Autodesk Inventor part; units mm, degrees
ref_plane "YZ Plane" through (0, 0, 0) normal (1, 0, 0) x (0, 1, 0)
ref_plane "XZ Plane" through (0, 0, 0) normal (0, 1, 0) x (-1, 0, 0)
ref_plane "XY Plane" through (0, 0, 0) normal (0, 0, 1) x (1, 0, 0)
sketch "Sketch1" plane through (0, 0, 0) normal (0, 0, 1) x (1, 0, 0)
  line L0 (0, 0) -> (38.1, 0)
  line L1 (38.1, 0) -> (38.1, 253.0348)
  arc A0 (38.1, 507.0348) -> (38.1, 253.0348) centre (666.75, 380.0348) ccw
  line L2 (38.1, 507.0348) -> (38.1, 608.6348)
  line L3 (38.1, 608.6348) -> (0, 608.6348)
  line L4 (0, 608.6348) -> (0, 0)
  circle A1 centre (31.75, 151.4348) radius 3.3655
  circle A2 centre (31.75, 34.671) radius 3.3655
  circle A3 centre (12.7, 12.7) radius 3.3655
  circle A4 centre (12.7, 342.9) radius 3.3655
  circle A5 centre (12.7, 595.9348) radius 3.3655
  circle A6 centre (31.75, 12.7) radius 3.3655
  circle A7 centre (31.75, 253.0348) radius 3.3655
  circle A8 centre (31.75, 507.0348) radius 3.3655
  circle A9 centre (31.75, 595.9348) radius 3.3655
  line L5 (0, 557.8348) -> (0, 608.6348)
  line L6 (0, 50.8) -> (0, 0)
  line L7 (12.7, 342.9) -> (0, 304.3174) construction
  line L8 (0, 317.5) -> (0, 368.3)
  line L9 (0, 129.921) -> (12.7, 129.921) construction
  circle A10 centre (12.7, 129.921) radius 3.3655
  circle A11 centre (12.7, 174.371) radius 3.3655
  line L10 (9.3413, 197.482) -> (9.3413, 204.213)
  line L11 (16.0611, 204.488) -> (16.0611, 197.3435)
  arc A12 (16.0611, 204.488) -> (9.3413, 204.213) centre (12.6956, 204.488) ccw
  arc A13 (9.3413, 197.482) -> (16.0611, 197.3435) centre (12.6974, 197.231) ccw
  circle A14 centre (12.7, 217.188) radius 3.3655
  dimension "d0" = 38.1
  dimension "d2" = 101.6
  dimension "d4" = 457.2
  dimension "d5" = 101.6
  dimension "d6" = 666.75
  dimension "d7" = 641.35
  dimension "d9" = 116.7638
  dimension "d10" = 6.35
  dimension "d11" = 6.35
  dimension "d13" = 12.7
  dimension "d14" = 12.7
  dimension "d16" = 12.7
  dimension "d17" = 342.9
  dimension "d19" = 12.7
  dimension "d20" = 12.7
  dimension "d22" = 6.35
  dimension "d24" = 6.35
  dimension "d25" = 6.731
  dimension "d26" = 6.35
  dimension "hole" = 6.731
  dimension "d28" = 6.35
  dimension "d45" = 12.7
  dimension "d47" = 12.7
  dimension "d54" = 6.731
  dimension "d55" = 3.3655
  dimension "d56" = 3.3655
  dimension "d58" = 6.731
  dimension "d59" = 12.7
  dimension "d68" = 18.22
  dimension "d69" = 90
  dimension "d70" = 90
  dimension "d71" = 22.0389
  dimension "d72" = 28.7587
  dimension "d73" = 478.7138
  dimension "d74" = 6.35
  dimension "d75" = 6.35
  dimension "d76" = 595.9348
  dimension "d77" = 404.1468
  dimension "d78" = 411.2913
  dimension "d79" = 25.4
  dimension "d80" = 25.4
  dimension "d81" = 434.2638
  dimension "d82" = 50.8
  dimension "d83" = 240.3348
  dimension "d84" = 291.1348
  dimension "d85" = 557.8348
extrude "Plate4" add sketch "Sketch1" along normal blind 3.048
sketch "Sketch5" plane through (0, 0, 3.048) normal (0, 0, 1) x (1, 0, 0)
  line L0 (38.1, 0) -> (38.1, 253.0348)
  line L1 (0, 0) -> (38.1, 0)
  line L2 (38.1, 0) -> (38.1, 25.4)
  line L3 (38.1, 25.4) -> (0, 25.4)
  line L4 (0, 25.4) -> (0, 0)
  dimension "d96" = 25.4
extrude "Cut1" cut sketch "Sketch5" against normal blind 3.048
sketch "Sketch7" plane through (0, 25.4, 3.048) normal (-1, 0, 0) x (0, -1, 0)
  line L0 (-583.2348, 0) -> (0, 0)
  line L1 (0, 0) -> (0, 22.352)
  line L2 (0, 22.352) -> (-583.2348, 22.352)
  line L3 (-583.2348, 22.352) -> (-583.2348, 0)
edge flange "Flange3" height 25.4 angle 90 thickness 3.048 bend radius 3.048 thickness toward (-1, 0, 0) relief tear relief width 3.048 relief depth 1.524 edges at (0, 317.0174, 3.048) wall of the first edge with corners at (0, 608.6348, 3.048) (0, 25.4, 3.048) (0, 25.4, 25.4) (0, 608.6348, 25.4)
bend "Bend3"
corner "Corner3"
sketch "Sketch8" plane through (38.1, 608.6348, 3.048) normal (0, 1, 0) x (1, 0, 0)
  line L0 (-41.148, -22.352) -> (0, -22.352)
  line L1 (0, -22.352) -> (0, 3.048)
  line L2 (0, 3.048) -> (-41.148, 3.048)
  line L3 (-41.148, 3.048) -> (-41.148, -22.352)
  point P0 (-38.1, 3.048)
extrude "Extrusion1" cut sketch "Sketch8" against normal blind 526.0848
equation "\"d25\" = hole"
equation "\"d97\" = Thickness"
equation "\"d109\" = BendReliefWidth"
equation "\"d110\" = BendReliefDepth"
equation "\"d111\" = MinimumRemnant"
equation "\"d112\" = BendRadius"
equation "\"d115\" = BendRadius"
equation "\"d116\" = CornerReliefSize"
equation "\"d117\" = GapSize"
equation "\"d118\" = JacobiRadiusSize"
equation "\"BendRadius\" = Thickness"
equation "\"BendReliefWidth\" = Thickness"
equation "\"BendReliefDepth\" = 0.5 * Thickness"
equation "\"CornerReliefSize\" = 4 * Thickness"
equation "\"MinimumRemnant\" = 2 * Thickness"
equation "\"TransitionRadius\" = BendRadius"
equation "\"JacobiRadiusSize\" = BendRadius"
equation "\"GapSize\" = Thickness"
equation "\"d29\" = BendRadius"
equation "\"d32\" = BendRadius"
equation "\"d38\" = BendRadius"
equation "\"d60\" = BendRadius"
properties part number "Claw - Arm - Top (R) v3"
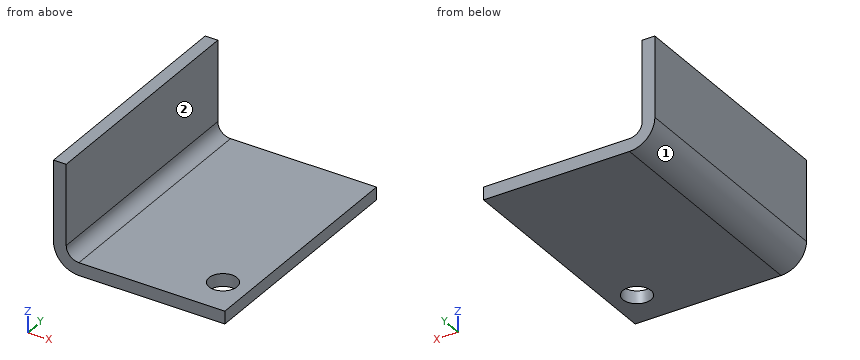
Build history of the part. All positions in model axes, mm. Face numbers are marked on the shaded views. A direction names the side the tool comes from. Round coordinates to 2 decimals unless told otherwise and drop trailing zeros. Loops run counter-clockwise (first coordinate to the right, second up) from the corner with the lowest first, then second, coordinate; pieces in that order, holes last.
Item 1: Which spindle directions (+Z, -Z, +X, -X, +Y, -Y) get a long thin tool onto all of the face, cutting with end or side? Do the marked faces 1 and 2. Say none if no direction does.
Item 2: Drill centre lines: line 1 along Y through (x, z) = (31.75, 2.1); line 2 along Z through (x, y) = (4, 68.5); line 3 along X through (y, z) = (30, 14.75). Where is each one in solid material? Low to high.
Item 3: Saw through at A-A (x = 31.75). List the corners of the cut face in (y, z), then the cut area to 3 significant figures.
Item 4: Pin check, flat tips, straight feed: P1, Ø12, axis at x = 20.5, y = 43.5, coming from the +Z side; P2, Ø2, axis at y = 52.5, z = 22.5, coming from the +X side. Stop position of each tip, or through.
Item 5: Saw through at C-C (z = 23). List the corners of the cut face in (x, y).
Item 6: Saw through at B-B (y = 36). List the corners of the cut face in (x, z).
Item 7: Saw through at D-D (y = 50). List the corners of the cut face in (x, z).
Worked answers:
1. face 1: -Z, -X, +Y, -Y
1. face 2: +Z, +X, +Y, -Y
2. line 1: y = 25.4 to 31.31, 38.04 to 82.55
2. line 2: z = 0 to 3.05
2. line 3: x = -3.05 to 0
3. outline: (25.4, 0) - (31.31, 0) - (31.31, 3.05) - (25.4, 3.05) - close; (38.04, 0) - (82.55, 0) - (82.55, 3.05) - (38.04, 3.05) - close
3. area: 154 mm2
4. P1: stops at z = 3.05
4. P2: stops at x = 0
5. outline: (-3.05, 25.4) - (0, 25.4) - (0, 82.55) - (-3.05, 82.55) - close
6. outline: (-3.05, 6.1) arc R6.1 ccw to (3.05, 0) - (28.66, 0) - (28.66, 3.05) - (3.05, 3.05) arc R3.05 cw to (0, 6.1) - (0, 25.4) - (-3.05, 25.4) - close; (34.84, 0) - (38.1, 0) - (38.1, 3.05) - (34.84, 3.05) - close
7. outline: (-3.05, 6.1) arc R6.1 ccw to (3.05, 0) - (38.1, 0) - (38.1, 3.05) - (3.05, 3.05) arc R3.05 cw to (0, 6.1) - (0, 25.4) - (-3.05, 25.4) - close
